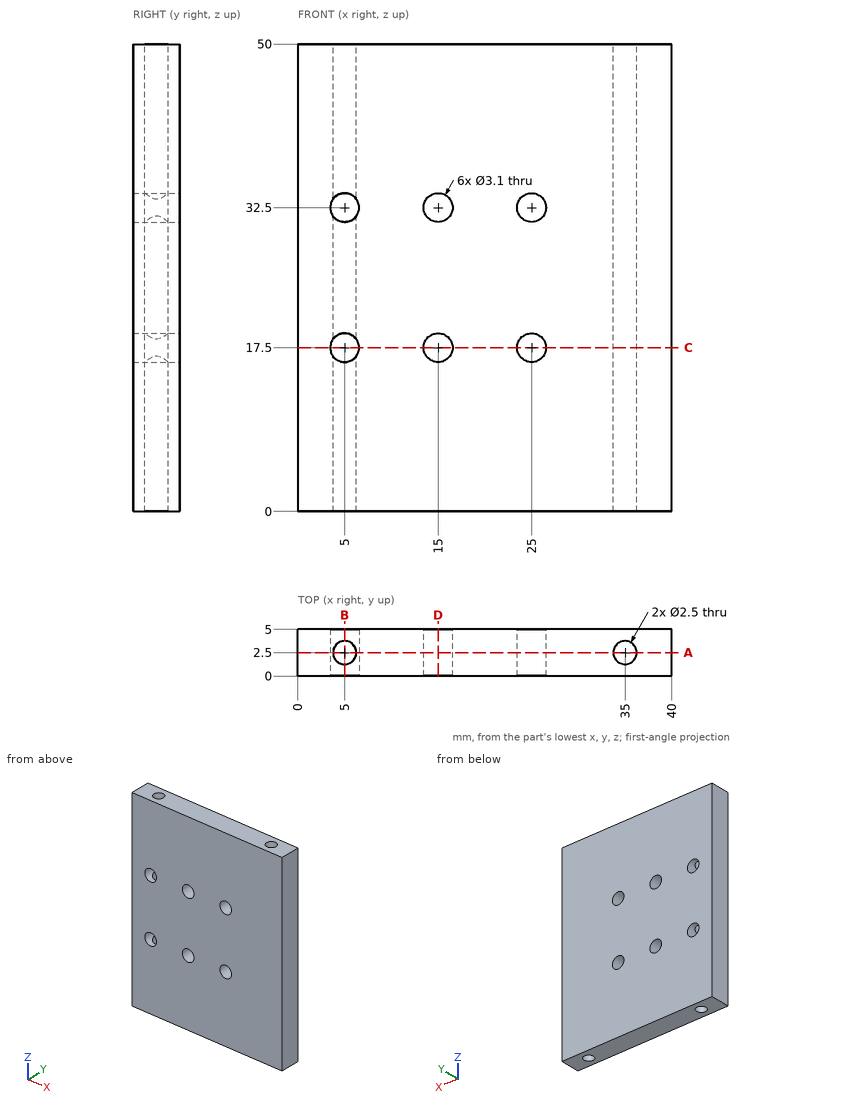
Study the drawing (mm; zero at the part's minimum x, y, z) and answer. Coordinates: 2 decimals unless noted, no trailing zeros. Write each loop counter-clockwise with the first axis right and the second up, starting at its lowest first coordinate (ties: lowest second). Pieces come first, ordered by that corner, then holes. Notation, with made-up numbers: (25, -35) - (57, -35) arc R32 cw to (57, -7) - close; hole circle Ø4 at (76.5, 2). An arc over 180 degrees is marked (long way). Put each result on its own line as item: value.
1. The part is cut by section B-B on x = 5. Give the vertices of the cut face in (y, z), plus the area to 4 significant figures.
Answer sheet:
outline: (0, 0) - (1.25, 0) - (1.25, 15.95) - (0, 15.95) - close; (0, 19.05) - (1.25, 19.05) - (1.25, 30.95) - (0, 30.95) - close; (0, 34.05) - (1.25, 34.05) - (1.25, 50) - (0, 50) - close; (3.75, 0) - (5, 0) - (5, 15.95) - (3.75, 15.95) - close; (3.75, 19.05) - (5, 19.05) - (5, 30.95) - (3.75, 30.95) - close; (3.75, 34.05) - (5, 34.05) - (5, 50) - (3.75, 50) - close
area: 109.5 mm^2
2. The part is cut by section C-C on z = 17.5. Give the vertices of the cut face in (x, y), plus the area to 3 significant figures.
Answer sheet:
outline: (0, 0) - (3.45, 0) - (3.45, 5) - (0, 5) - close; (6.55, 0) - (13.45, 0) - (13.45, 5) - (6.55, 5) - close; (16.55, 0) - (23.45, 0) - (23.45, 5) - (16.55, 5) - close; (26.55, 0) - (40, 0) - (40, 5) - (26.55, 5) - close; hole circle Ø2.5 at (35, 2.5)
area: 149 mm^2
3. The part is cut by section A-A on y = 2.5. Give the vertices of the cut face in (x, z).
Answer sheet:
outline: (0, 0) - (3.75, 0) - (3.75, 16.58) arc R1.55 cw to (3.75, 18.42) - (3.75, 31.58) arc R1.55 cw to (3.75, 33.42) - (3.75, 50) - (0, 50) - close; (6.25, 0) - (33.75, 0) - (33.75, 50) - (6.25, 50) - (6.25, 33.42) arc R1.55 cw to (6.25, 31.58) - (6.25, 18.42) arc R1.55 cw to (6.25, 16.58) - close; (36.25, 0) - (40, 0) - (40, 50) - (36.25, 50) - close; hole circle Ø3.1 at (15, 17.5); hole circle Ø3.1 at (15, 32.5); hole circle Ø3.1 at (25, 17.5); hole circle Ø3.1 at (25, 32.5)
4. The part is cut by section D-D on x = 15. Give the vertices of the cut face in (y, z), plus the area to 3 significant figures.
Answer sheet:
outline: (0, 0) - (5, 0) - (5, 15.95) - (0, 15.95) - close; (0, 19.05) - (5, 19.05) - (5, 30.95) - (0, 30.95) - close; (0, 34.05) - (5, 34.05) - (5, 50) - (0, 50) - close
area: 219 mm^2
5. Find the intervals of material crossed by line 1 along X through (y, z) = (2.5, 35.5); line 2 along Z through (x, y) = (25, 1.35); line 3 along Y through (x, z) = (5, 43), in increasing order. Write a range as from..to.
Answer sheet:
line 1: x = 0..3.75, 6.25..33.75, 36.25..40
line 2: z = 0..15.95, 19.05..30.95, 34.05..50
line 3: y = 0..1.25, 3.75..5
